Here's how the part is built. I have some questions about the finished solid (model axes, mm). Round coordinates to 2 decimals unless told otherwise and drop trailing zeros. Order: outer loops, then holes, each group sorted by start corner. A loop starts at its lowest first (then second) coordinate and runs counter-clockwise, first axis right, second up. Notation, with made-up numbers: M 7,-23.5 L 13,-23.5 A20 ccw 13,11.5 Z; hole C -2.75,63 d4. An arc over 180 degrees is marked long. Write item = value, one per line. Start each with the question number.
Item 1: Please list where these lines run through material, in increasing order: L1, parallel to Z at x = 2.45, y = -125; L2, parallel to Z at x = 3.3, y = 5; L3, parallel to Y at x = 2.45, z = 258.5.
Item 2: I'm going to push flat-ended pins straight in: P1, Ø1.8, axis at x = 3.5, z = 265, coming from the -Y side; P2, Ø1.8, axis at x = 1.5, y = -63, coming from the -Z side; P3, Ø1.8, axis at x = 2.5, z = 231, coming from the -Y side; P4, Ø5, axis at y = -125, z = 260, coming from the +X side. Where does each tip first touch, or does it pass through?
Item 3: I want a section at B-B, the plane x = 4.9. List the corners of the cut face in (y, z) for me.
Item 4: I want a section at C-C, the plane y = -61.5. List the corners of the cut face in (x, z) for me, plus the area to 3 significant figures.
Item 5: I want a section at A-A, the plane y = -125. List the corners of the cut face in (x, z) for me, plus the area to 3 significant figures.
```python
from build123d import *

# Parameters (mm, degrees)
F0_R     = 2
F1_DEPTH = 6


with BuildPart() as f1:
    # F0 (on Right) → F1 (new body)
    with BuildSketch(Plane.YZ):
        with BuildLine():
            Line((-150, 250), (-1.27, 250))
            ThreePointArc((-1.27, 250), (-0.371974, 249.628026), (0, 248.73))
            Line((0, 248.73), (0, 240))
            Line((0, 240), (10, 240))
            Line((10, 240), (10, 225))
            Line((10, 225), (20, 225))
            Line((20, 225), (20, 270))
            Line((20, 270), (-135, 270))
            Line((-135, 270), (-135, 260))
            Line((-135, 260), (-150, 260))
            Line((-150, 260), (-150, 250))
        make_face()
        with Locations((-125, 260)):
            Circle(F0_R, mode=Mode.SUBTRACT)
        with Locations((10, 260)):
            Circle(F0_R, mode=Mode.SUBTRACT)
    extrude(amount=F1_DEPTH)


solid = f1.part
```
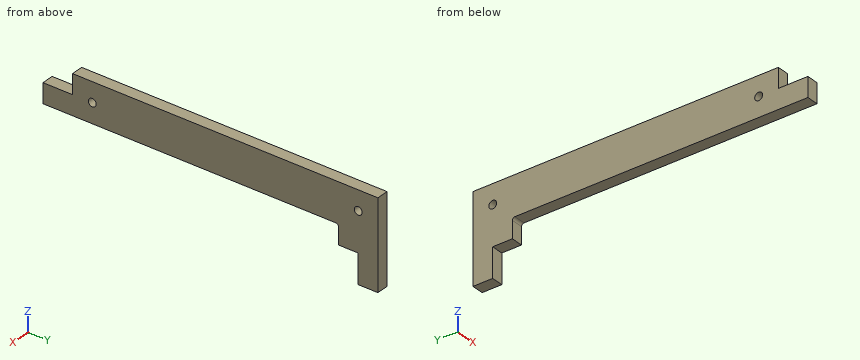
Filled in:
q1.L1 = 250 to 258, 262 to 270
q1.L2 = 240 to 270
q1.L3 = -150 to -126.32, -123.68 to 8.68, 11.32 to 20
q2.P1 = -135
q2.P2 = 250
q2.P3 = 10
q2.P4 = 6
q3.outline = M -150,250 L -1.27,250 A1.27 cw 0,248.73 L 0,240 L 10,240 L 10,225 L 20,225 L 20,270 L -135,270 L -135,260 L -150,260 Z; hole C -125,260 d4; hole C 10,260 d4
q4.outline = M 0,250 L 6,250 L 6,270 L 0,270 Z
q4.area = 120 mm^2
q5.outline = M 0,250 L 6,250 L 6,258 L 0,258 Z; M 0,262 L 6,262 L 6,270 L 0,270 Z
q5.area = 96.0 mm^2
